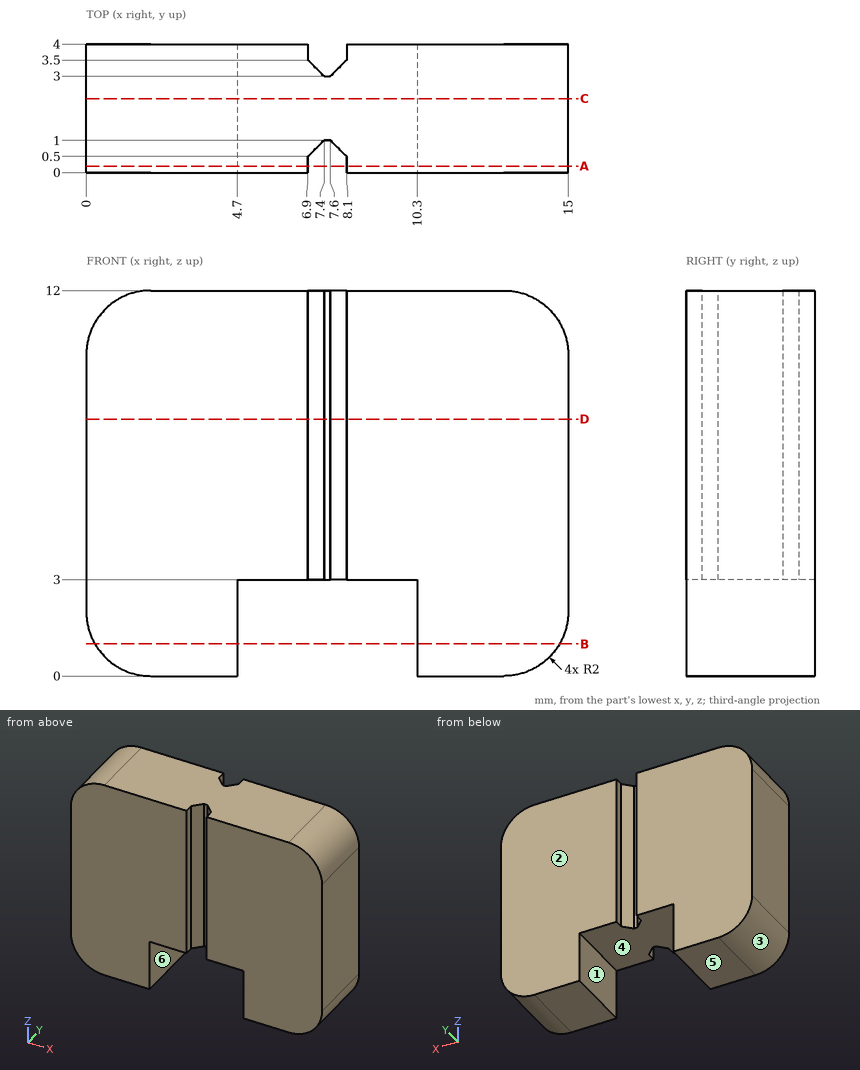
Geometry: see drawing. Coordinates: mm, zero at the bounding-box minimum. A direction names the side the tool comes from. Give positions to 0.01 mm unless a question says otherwise; leave off trailing zeros. Write each loop counter-clockwise with the first axis right and the second up, starting at its lowest first coordinate (ties: lowest second). Pieces come first, ordered by that corner, then holes. Notation, with made-up numbers: M -11,62.5 L 40,62.5 A19 cw 40,66.5 Z; hole C -2.75,-35 d7. An arc over 180 degrees is marked long. Answer as a JSON object with one key per item and string values.
Q1. Cut plane C-C, the plane y = 2.3. Return the cut outline in (x, z).
Geometry check:
{"outline": "M 0,2 A2 ccw 2,0 L 4.7,0 L 4.7,3 L 10.3,3 L 10.3,0 L 13,0 A2 ccw 15,2 L 15,10 A2 ccw 13,12 L 2,12 A2 ccw 0,10 Z"}
Q2. Mould query, pull axis X, two halves, no side actions, for the marked faces 1, 2, 3 and 4. Classes: +X half, -X half, draft (parallel to the pull), parting line (faces both ways), or undercut.
Geometry check:
{"face 1": "undercut", "face 2": "draft", "face 3": "-X half", "face 4": "undercut"}
Q3. Cut plane B-B, the plane z = 1. Return the cut outline in (x, y), then the cut area to 3 significant figures.
Geometry check:
{"outline": "M 0.27,0 L 4.7,0 L 4.7,4 L 0.27,4 Z; M 10.3,0 L 14.73,0 L 14.73,4 L 10.3,4 Z", "area": "35.5 mm^2"}
Q4. Access query for the marked faces 5 and 6. Directions: +Z, -Z, +X, -X, +Y, -Y. A direction counts if a zero-diameter tool reaches every point of the face in a straight line with its end or side. Return the directions, or none.
Geometry check:
{"face 5": "-Z, +X, -X, +Y, -Y", "face 6": "-Z, +Y, -Y"}
Q5. Ray query, line 1 along X through (y, z) = (1.95, 2.25); line 2 along Z through (x, y) = (9, 1); line 3 along X through (y, z) = (0.9, 7.75). Return the intervals inside material, ascending.
Geometry check:
{"line 1": "x = 0 to 4.7, 10.3 to 15", "line 2": "z = 3 to 12", "line 3": "x = 0 to 7.3, 7.7 to 15"}
Q6. Cut plane A-A, the plane y = 0.2. Return the cut outline in (x, z).
Geometry check:
{"outline": "M 0,2 A2 ccw 2,0 L 4.7,0 L 4.7,3 L 6.9,3 L 6.9,12 L 2,12 A2 ccw 0,10 Z; M 8.1,3 L 10.3,3 L 10.3,0 L 13,0 A2 ccw 15,2 L 15,10 A2 ccw 13,12 L 8.1,12 Z"}
Q7. Contact query for a flat-ended pin moving along its axis: P1, Ø1, axis at x = 5, y = 2, coming from the -Z side. Output: stop coordinate, or through.
Geometry check:
{"P1": "stops at z = 0"}
Q8. Cut plane D-D, the plane z = 8. Return the cut outline in (x, y), then the cut area to 3 significant figures.
Geometry check:
{"outline": "M 0,0 L 6.9,0 L 6.9,0.5 L 7.4,1 L 7.6,1 L 8.1,0.5 L 8.1,0 L 15,0 L 15,4 L 8.1,4 L 8.1,3.5 L 7.6,3 L 7.4,3 L 6.9,3.5 L 6.9,4 L 0,4 Z", "area": "58.1 mm^2"}
